```python
from build123d import *

# Parameters (mm, degrees)
SKETCH1_R           = 14
SKETCH1_R_2         = 1.5
BOSS_EXTRUDE1_DEPTH = 3


with BuildPart() as part:
    # Sketch1 → Boss-Extrude1 (new body)
    with BuildSketch(Plane(origin=(0, 0, 0), x_dir=(1, 0, 0), z_dir=(0, 1, 0))):
        Circle(SKETCH1_R)
        with Locations((-4.324322786, -10.439838717)):
            Circle(SKETCH1_R_2, mode=Mode.SUBTRACT)
        with Locations((10.439838717, -4.324322786)):
            Circle(SKETCH1_R_2, mode=Mode.SUBTRACT)
        with Locations((4.324322786, 10.439838717)):
            Circle(SKETCH1_R_2, mode=Mode.SUBTRACT)
        with Locations((-10.439838717, 4.324322786)):
            Circle(SKETCH1_R_2, mode=Mode.SUBTRACT)
        with BuildLine():
            ThreePointArc((-3.820621038, -3.956368902), (-2.060336264, -5.0995112), (0, -5.5))
            Line((0, -5.5), (0, -8.6))
            ThreePointArc((0, -8.6), (3.360287705, -7.91634174), (6.186322283, -5.974061986))
            Line((6.186322283, -5.974061986), (3.956368902, -3.820621038))
            ThreePointArc((3.956368902, -3.820621038), (5.0995112, -2.060336264), (5.5, 0))
            Line((5.5, 0), (8.6, 0))
            ThreePointArc((8.6, 0), (7.91634174, 3.360287705), (5.974061986, 6.186322283))
            Line((5.974061986, 6.186322283), (3.820621038, 3.956368902))
            ThreePointArc((3.820621038, 3.956368902), (2.060336264, 5.0995112), (0, 5.5))
            Line((0, 5.5), (0, 8.6))
            ThreePointArc((0, 8.6), (-3.360287705, 7.91634174), (-6.186322283, 5.974061986))
            Line((-6.186322283, 5.974061986), (-3.956368902, 3.820621038))
            ThreePointArc((-3.956368902, 3.820621038), (-5.0995112, 2.060336264), (-5.5, 0))
            Line((-5.5, 0), (-8.6, 0))
            ThreePointArc((-8.6, 0), (-7.91634174, -3.360287705), (-5.974061986, -6.186322283))
            Line((-5.974061986, -6.186322283), (-3.820621038, -3.956368902))
        make_face(mode=Mode.SUBTRACT)
    extrude(amount=BOSS_EXTRUDE1_DEPTH)


solid = part.part
```
Check sheet for the modelled part. Datum: model origin and axes. Units: mm. A direction names the side the tool comes from. Coordinates: 2 decimals unless noted, no trailing zeros. Order: outer loops, then holes, each group sorted by start corner. A loop starts at its lowest first (then second) coordinate and runs counter-clockwise, first axis right, second up. Notation, with made-up numbers: M -31,-38 L -13,-38 A11 ccw -13,-25 Z; hole C 78,53 d4. An arc over 180 degrees is marked long. One line per question, with ' | ' between items. Start each with the question number.
Item 1: Gauge pin test, flat ends, axial feed: P1, Ø0.9, axis at x = -7, y = 2, coming from the +Z side; P2, Ø4, axis at x = -4.32, z = 10.44, coming from the -Y side; P3, Ø0.9, axis at x = 7.5, y = 1.5, coming from the -Z side; P4, Ø1, axis at y = 2.5, z = 5, coming from the -X side. Record the tip position at first contact, or that the pin passes through.
Item 2: Mould release check, pull along Z, two halves, no side actions. Record for faces 1 (the flat face through (-5.087, 1.479, -4.912)), 2 (the flat face through (-0.2, 0, 6)), 3 (the cylindrical face through (12.932, 1.479, 5.362)): pulls with the +Z half, pulls with the -Z half, needs draft (parallel to the pull), parting line crosses it, or undercut.
Item 3: Sectioned sample at C-C on z = 6.75. Record the cut outline in (x, y), and give its area (3 significant figures).
Item 4: Sectioned sample at A-A on y = 1.05. Record the cut outline in (x, z).
Item 5: Material ranges on line 1 (X direction, y = 1.45, z = 4.75); line 2 (Z direction, x = 0.25, y = 1.55); line 3 (X direction, y = 2.2, z = -4.5), recorded low to high.
Item 6: Access from +Z, -Z, +X, -X, +Y, -Y to the whole of each face (thin tool, end or side, straight path). Record for faces 4 (the flat face through (-0.2, 3, 6)), 5 (the flat face through (0, 1, -7)).
Item 7: Sectioned sample at B-B on z = 1. Record the cut outline in (x, y), and give its area (3 significant figures).
Answer below:
1) P1: stops at z = 12.37 | P2: stops at y = 0 | P3: stops at z = -12.1 | P4: stops at x = -13.26
2) face 1: undercut | face 2: needs draft | face 3: parting line crosses it
3) outline: M -12.27,0 L 0,0 L 0,3 L -12.27,3 Z; M 5.33,0 L 12.27,0 L 12.27,3 L 5.33,3 Z | area: 57.6 mm^2
4) outline: C 0,0 d28; hole C -10.44,-4.32 d3; hole M -8.6,0 L -5.5,0 A5.5 ccw -3.96,-3.82 L -6.19,-5.97 A8.6 ccw 0,-8.6 L 0,-5.5 A5.5 ccw 3.82,-3.96 L 5.97,-6.19 A8.6 ccw 8.6,0 L 5.5,0 A5.5 ccw 3.96,3.82 L 6.19,5.97 A8.6 ccw 0,8.6 L 0,5.5 A5.5 ccw -3.82,3.96 L -5.97,6.19 A8.6 ccw Z; hole C -4.32,10.44 d3; hole C 4.32,-10.44 d3; hole C 10.44,4.32 d3
5) line 1: x = -13.17 to -7.17, -4.59 to -2.77, 4.92 to 9, 11.88 to 13.17 | line 2: z = -14 to -5.49, 8.6 to 14 | line 3: x = -13.26 to -11.93, -8.95 to -4.66, 3.16 to 4.35, 7.33 to 13.26
6) face 4: +Z, -Z, +X, -X, +Y | face 5: +Y, -Y
7) outline: M -13.96,0 L -8.54,0 L -8.54,3 L -13.96,3 Z; M 5.41,0 L 13.96,0 L 13.96,3 L 5.41,3 Z | area: 41.9 mm^2
